Could you check a few things on this model? Use its own coordinates, in mm. Face numbers are marked on the shaded views. A direction names the side the tool comes from. Give positions to 0.01 mm unless a question says otherwise; leave off trailing zeros. Write each loop counter-clockwise with the first axis right and the second up, starting at its lowest first coordinate (ties: lowest second). Pieces come first, ordered by that corner, then holes. Notation, with made-up numbers: (28.25, 38) - (51.25, 38) arc R19 ccw to (51.25, 64) - close; hole circle Ø5 at (-10, 10.5). An arc over 180 degrees is marked (long way). Write item = value, one per line.
from build123d import *

# Parameters (mm, degrees)
F0_W     = 25
F0_H     = 30
F1_DEPTH = 3
F2_W     = 25
F2_H     = 2.5
F3_DEPTH = 3
F4_W     = 4
F4_H     = 13.7322908992
F5_DEPTH = 15
F6_R     = 2
F7_W     = 8
F7_H     = 8
F8_DEPTH = 3


with BuildPart() as f1:
    # F0 (on Top) → F1 (new body)
    with BuildSketch(Plane.XY):
        Rectangle(F0_W, F0_H)
    extrude(amount=F1_DEPTH)

    # F2 (on face) → F3 (join)
    with BuildSketch(Plane.XY.offset(3)):
        with Locations((0, 13.75)):
            Rectangle(F2_W, F2_H)
        with Locations((0, -13.75)):
            Rectangle(F2_W, F2_H)
    extrude(amount=F3_DEPTH)

    # F4 (on Top) → F5 (join)
    with BuildSketch(Plane.XY):
        with Locations((-14.5, 0)):
            Rectangle(F4_W, F4_H)
    extrude(amount=F5_DEPTH)

    # F6
    f6_edges = [f1.edges().sort_by_distance(p)[0] for p in [
        (-12.5, -6.866145, 1.5),
        (-12.5, 6.866145, 1.5),
    ]]
    fillet(f6_edges, radius=F6_R)

    # F7 (on face) → F8 (cut)
    with BuildSketch(Plane.XY.offset(3)):
        with Locations((-6.25, 6.25)):
            Rectangle(F7_W, F7_H)
        with Locations((6.25, 6.25)):
            Rectangle(F7_W, F7_H)
        with Locations((-6.25, -6.25)):
            Rectangle(F7_W, F7_H)
        with Locations((6.25, -6.25)):
            Rectangle(F7_W, F7_H)
    extrude(amount=-F8_DEPTH, mode=Mode.SUBTRACT)


solid = f1.part
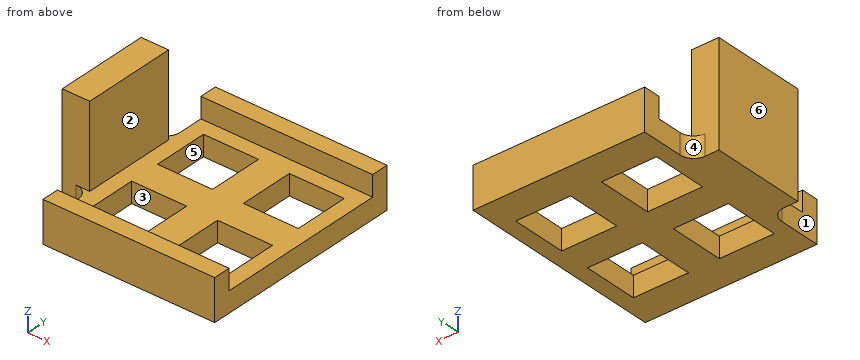
1. Thinking about a two-plate mould opening in Y: for the marked faces 4, 5 and 6, which applies, pulls with the +Y half, pulls with the -Y half, needs draft (parallel to the pull), parting line crosses it, or undercut?
Filled sheet:
face_4 = pulls with the +Y half
face_5 = undercut
face_6 = needs draft
2. If we section it at D-D, the plane y = 9.25: Please give me the cut outline in (x, z), and give its area (3 significant figures).
Filled sheet:
outline = (-12.5, 0) - (-10.25, 0) - (-10.25, 3) - (-12.5, 3) - close; (-2.25, 0) - (2.25, 0) - (2.25, 3) - (-2.25, 3) - close; (10.25, 0) - (12.5, 0) - (12.5, 3) - (10.25, 3) - close
area = 27.0 mm2
3. If we section it at C-C, the plane x = 5: Please give me the cut outline in (y, z), and give its area (3 significant figures).
Filled sheet:
outline = (-15, 0) - (-10.25, 0) - (-10.25, 3) - (-12.5, 3) - (-12.5, 6) - (-15, 6) - close; (-2.25, 0) - (2.25, 0) - (2.25, 3) - (-2.25, 3) - close; (10.25, 0) - (15, 0) - (15, 6) - (12.5, 6) - (12.5, 3) - (10.25, 3) - close
area = 57.0 mm2
4. Which directions (+Z, -Z, +X, -X, +Y, -Y) give clear straight access to the entire face, cutting with the end or side of a thin tool? Please do the marked faces 1, 2 and 3.
Filled sheet:
face_1 = +Z, -Z, -X, -Y
face_2 = +Z, +X
face_3 = +Z, -Z
5. If we section it at A-A, the plane z = 4.75: Please give me the cut outline in (x, y).
Filled sheet:
outline = (-16.5, -6.87) - (-12.5, -6.87) - (-12.5, 6.87) - (-16.5, 6.87) - close; (-12.5, -15) - (12.5, -15) - (12.5, -12.5) - (-12.5, -12.5) - close; (-12.5, 12.5) - (12.5, 12.5) - (12.5, 15) - (-12.5, 15) - close
6. I need wall thicknesses on line 1 (Y direction, x = 3, z = 2); line 2 (X direction, y = -2.5, z = 0.5); line 3 (X direction, y = -9, z = 1). Which ranges of each line are inside material? Lowest first, please.
Filled sheet:
line_1 = -15 to -10.25, -2.25 to 2.25, 10.25 to 15
line_2 = -16.5 to -10.25, -2.25 to 2.25, 10.25 to 12.5
line_3 = -12.5 to -10.25, -2.25 to 2.25, 10.25 to 12.5
7. If we section it at B-B, the plane y = 3.75: Please give me the cut outline in (x, z), and give its area (3 significant figures).
Filled sheet:
outline = (-16.5, 0) - (-10.25, 0) - (-10.25, 3) - (-12.5, 3) - (-12.5, 15) - (-16.5, 15) - close; (-2.25, 0) - (2.25, 0) - (2.25, 3) - (-2.25, 3) - close; (10.25, 0) - (12.5, 0) - (12.5, 3) - (10.25, 3) - close
area = 87.0 mm2
8. For pin 1 (2 mm diameter, centred on x = 2, y = 13, fed in from +Z); pin 2 (2 mm diameter, centred on x = -15.5, z = 10.5, fed in from -Y); pin 3 (1.5 mm diameter, centred on y = 4, z = 7.5, fed in from +X), each with a flat end and sliding along its axis, tell me the tip position at first contact or that it passes through.
Filled sheet:
pin_1 = 6
pin_2 = -6.87
pin_3 = -12.5
